```python
from build123d import *

# Parameters (mm, degrees)
BOSS_EXTRUDE1_DEPTH      = 20
BOSS_EXTRUDE1_DEPTH_BACK = 20
SKETCH1_W                = 20
SKETCH1_H                = 2
BOSS_EXTRUDE2_DEPTH      = 7
BOSS_EXTRUDE2_DEPTH_BACK = 7
SKETCH3_W                = 7
SKETCH3_H                = 15
CUT_EXTRUDE1_DEPTH       = 60
FILLET1_R                = 2
SKETCH4_R                = 3.5
CUT_EXTRUDE2_DEPTH       = 60
FILLET3_R                = 2


with BuildPart() as part:
    # Sketch1 → Boss-Extrude1 (new, two sides: drawn at the far end of the back side and taken through both)
    with BuildSketch(Plane.XY.offset(-BOSS_EXTRUDE1_DEPTH_BACK)):
        with BuildLine():
            ThreePointArc((10, 0), (0, -4.202041029), (-10, 0))
            Line((-10, 0), (10, 0))
        make_face()
        with Locations((0, 1)):
            Rectangle(SKETCH1_W, SKETCH1_H)
    extrude(amount=BOSS_EXTRUDE1_DEPTH + BOSS_EXTRUDE1_DEPTH_BACK)

    # Sketch2 → Boss-Extrude2 (add, two sides: drawn at the far end of the back side and taken through both)
    with BuildSketch(Plane(origin=(0, 0, 0), x_dir=(0, 0, -1), z_dir=(1, 0, 0)).offset(-BOSS_EXTRUDE2_DEPTH_BACK)):
        with BuildLine():
            ThreePointArc((7, 9.2), (0, 16.2), (-7, 9.2))
            Line((-7, 9.2), (-2.1, 9.2))
            ThreePointArc((-2.1, 9.2), (0, 11.3), (2.1, 9.2))
            Line((2.1, 9.2), (7, 9.2))
        make_face()
        with BuildLine():
            Line((-2.1, 9.2), (-7, 9.2))
            ThreePointArc((-7, 9.2), (0, 2.2), (7, 9.2))
            Line((7, 9.2), (2.1, 9.2))
            ThreePointArc((2.1, 9.2), (0, 7.1), (-2.1, 9.2))
        make_face()
        with BuildLine():
            Line((-7, 9.2), (-7, 2))
            Line((-7, 2), (7, 2))
            Line((7, 2), (7, 9.2))
            ThreePointArc((7, 9.2), (0, 2.2), (-7, 9.2))
        make_face()
    extrude(amount=BOSS_EXTRUDE2_DEPTH + BOSS_EXTRUDE2_DEPTH_BACK)

    # Sketch3 → Cut-Extrude1 (cut)
    with BuildSketch(Plane.XY.offset(7)):
        with Locations((0, 9.5)):
            Rectangle(SKETCH3_W, SKETCH3_H)
    extrude(amount=-CUT_EXTRUDE1_DEPTH, mode=Mode.SUBTRACT)

    # Fillet1
    fillet1_edges = [part.edges().sort_by_distance(p)[0] for p in [
        (-10, 0, 0),
        (10, 0, 0),
    ]]
    fillet(fillet1_edges, radius=FILLET1_R)

    # Sketch4 → Cut-Extrude2 (cut)
    with BuildSketch(Plane.XY.offset(20)):
        with Locations((0, 2)):
            Circle(SKETCH4_R)
    extrude(amount=-CUT_EXTRUDE2_DEPTH, mode=Mode.SUBTRACT)

    # Fillet3
    fillet3_edges = [part.edges().sort_by_distance(p)[0] for p in [
        (-7, 16.2, 0),
        (-7, 5.6, -7),
        (7, 5.6, 7),
        (-7, 5.6, 7),
        (7, 16.2, 0),
        (7, 5.6, -7),
    ]]
    fillet(fillet3_edges, radius=FILLET3_R)


solid = part.part
```
Part model, mm, in its own coordinate system. A direction names the side the tool comes from. Round coordinates to 2 decimals unless told otherwise and drop trailing zeros. Loops run counter-clockwise (first coordinate to the right, second up) from the corner with the lowest first, then second, coordinate; pieces in that order, holes last. Notation, with made-up numbers: (-27, -9.5) -> (-10, -9.5) arc R14 cw to (-10, 0.5) -> close; hole circle Ø8 at (62.25, -12). An arc over 180 degrees is marked (long way). Use a Markdown table: item, result.
1) Cut at A-A, the plane z = 0. List the corners of the cut face in (x, y).
The answers:
| item | result |
|---|---|
| outline | (-10, 0.85) arc R2 ccw to (-9.33, -0.64) arc R14 ccw to (9.33, -0.64) arc R2 ccw to (10, 0.85) -> (10, 2) -> (7, 2) -> (7, 7.1) -> (3.5, 7.1) -> (3.5, 2) arc R3.5 cw to (-3.5, 2) -> (-3.5, 7.1) -> (-7, 7.1) -> (-7, 2) -> (-10, 2) -> close; (-7, 11.3) -> (-3.5, 11.3) -> (-3.5, 16.2) -> (-5, 16.2) arc R2 ccw to (-7, 14.2) -> close; (3.5, 11.3) -> (7, 11.3) -> (7, 14.2) arc R2 ccw to (5, 16.2) -> (3.5, 16.2) -> close |
2) Tool access for faces 1 (the flat face through (4, 6, 7)), 2 (the flat face through (-8, 2, 0)), 3 (the cylindrical face through (-6.43, 5.55, 6.4)), 4 (the flat face through (-7, 6.8, 0.1)), 5 (the flat face through (-3.5, 7, 2)): list every direction of +Z, -Z, +X, -X, +Y, -Y with a clear straight run to the whole face (end or side of a thin tool).
The answers:
| item | result |
|---|---|
| face 1 | +Z, +X, -X, +Y |
| face 2 | -X, +Y |
| face 3 | +Z, -X, +Y |
| face 4 | +Z, -Z, -X, +Y |
| face 5 | +Z, -Z, +Y |
3) Cut at B-B, the plane x = -6.25. List the corners of the cut face in (y, z).
The answers:
| item | result |
|---|---|
| outline | (-2.73, -20) -> (2, -20) -> (2, -6.56) -> (9.2, -6.56) arc R6.56 ccw to (9.2, 6.56) -> (2, 6.56) -> (2, 20) -> (-2.73, 20) -> close; hole circle Ø4.2 at (9.2, 0) |
4) Cut at C-C, the plane x = 0. List the corners of the cut face in (y, z).
The answers:
| item | result |
|---|---|
| outline | (-4.2, -20) -> (-1.5, -20) -> (-1.5, 20) -> (-4.2, 20) -> close |
5) Drop flat-ended pins along their axis: pin 1 Ø4 at (y, z) = (6, 3) entering from -X; pin 2 Ø2 at (x, z) = (-6, -0.5) entering from +Y; pin 3 Ø1.6 at (x, y) = (-4, 4.5) entering from -Z. Give the stop position or say it passes through.
The answers:
| item | result |
|---|---|
| pin 1 | stops at x = -7 |
| pin 2 | stops at y = 16.2 |
| pin 3 | stops at z = -7 |
6) Pull direction Y, two halves, no side cores. Call faces 6 (the cylindrical face through (0.1, -4.2, -0.3)), 7 (the cylindrical face through (5.23, 11.25, 0.46)), 8 (the flat face through (10, 1.4, -0.3)): pulls with the +Y half, pulls with the -Y half, needs draft (parallel to the pull), parting line crosses it, or undercut.
The answers:
| item | result |
|---|---|
| face 6 | pulls with the -Y half |
| face 7 | undercut |
| face 8 | needs draft |
7) Cut at D-D, the plane y = -3. List the corners of the cut face in (x, z).
The answers:
| item | result |
|---|---|
| outline | (-5.68, -20) -> (5.68, -20) -> (5.68, 20) -> (-5.68, 20) -> close |
8) Probe line 1 (Z direction, x = -4.4, y = 9.2); line 2 (X direction, y = 7, z = 2); line 3 (X direction, y = 1, z = 15). List the from-to ranges inside material, lowest first. Write a range as [from, to].
The answers:
| item | result |
|---|---|
| line 1 | z = [-7, -2.1], [2.1, 7] |
| line 2 | x = [-7, -3.5], [3.5, 7] |
| line 3 | x = [-10, -3.35], [3.35, 10] |
